Here's how the part is built. I have some questions about the finished solid (model axes, mm). Coordinates: 2 decimals unless noted, no trailing zeros. Write each loop counter-clockwise with the first axis right and the second up, starting at its lowest first coordinate (ties: lowest second). Pieces come first, ordered by that corner, then holes.
```python
from build123d import *

# Parameters (mm, degrees)
F1_DEPTH = 1
F2_R     = 2
F3_R     = 2.4
F4_DEPTH = 25
F5_R     = 2


with BuildPart() as f1:
    # F0 (on Front) → F1 (new body, symmetric)
    with BuildSketch(Plane.XZ):
        with BuildLine():
            ThreePointArc((28.013159, -35.217367), (14.836079, -42.484006), (0, -45))
            ThreePointArc((0, -45), (-14.836079, -42.484006), (-28.013159, -35.217367))
            Line((-28.013159, -35.217367), (-35, -44.00103))
            Line((-35, -44.00103), (-35, -65))
            Line((-35, -65), (35, -65))
            Line((35, -65), (35, -44.00103))
            Line((35, -44.00103), (28.013159, -35.217367))
        make_face()
        with BuildLine():
            ThreePointArc((0, -50), (-15.45085, -47.552826), (-29.389263, -40.45085))
            Line((-29.389263, -40.45085), (-27.038122, -37.214782))
            ThreePointArc((-27.038122, -37.214782), (-14.214782, -43.7486), (0, -46))
            ThreePointArc((0, -46), (14.214782, -43.7486), (27.038122, -37.214782))
            Line((27.038122, -37.214782), (29.389263, -40.45085))
            ThreePointArc((29.389263, -40.45085), (15.45085, -47.552826), (0, -50))
        make_face(mode=Mode.SUBTRACT)
    extrude(amount=F1_DEPTH, both=True)

    # F2
    f2_edges = [f1.edges().sort_by_distance(p)[0] for p in [
        (28.013159, 0, -35.217367),
        (35, 0, -44.00103),
        (-28.013159, 0, -35.217367),
        (-35, 0, -44.00103),
    ]]
    fillet(f2_edges, radius=F2_R)

    # F3 (on face) → F4 (cut)
    with BuildSketch(Plane.XZ.offset(1)):
        with Locations((-25, -55)):
            Circle(F3_R)
        with Locations((25, -55)):
            Circle(F3_R)
    extrude(amount=-F4_DEPTH, mode=Mode.SUBTRACT)

    # F5
    f5_edges = [f1.edges().sort_by_distance(p)[0] for p in [
        (35, 0, -65),
        (-35, 0, -65),
    ]]
    fillet(f5_edges, radius=F5_R)


solid = f1.part
```
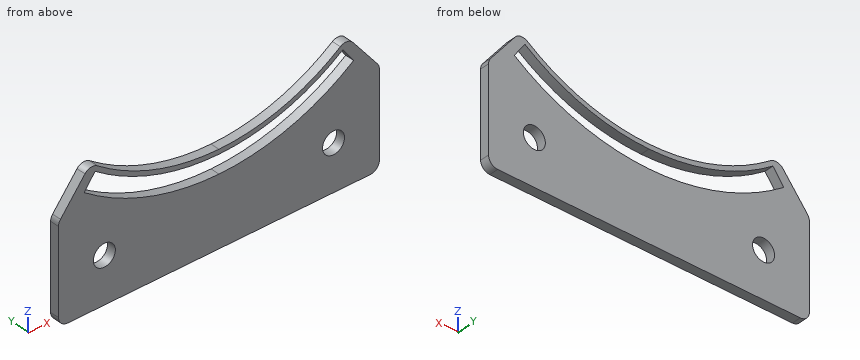
1) Imagine slicing it at A-A on z = -55. Please give me the cut outline in (x, y), then the cut area to 3 significant figures.
Values follow:
outline: (-35, -1) - (-27.4, -1) - (-27.4, 1) - (-35, 1) - close; (-22.6, -1) - (22.6, -1) - (22.6, 1) - (-22.6, 1) - close; (27.4, -1) - (35, -1) - (35, 1) - (27.4, 1) - close
area: 121 mm2
2) Will these pins go through, and if not, where does the flat tip stop? pin 1 (5.5 mm diameter, centred on x = -25, z = -55, fed in from -Y); pin 2 (1 mm diameter, centred on y = 0.5, z = -41, fed in from -X).
Values follow:
pin 1: stops at y = -1
pin 2: stops at x = -33.01
3) I need wall thicknesses on probe 1 along Z at (x, y) = (27, 0.2); probe 2 along X at (y, z) = (-0.45, -53.75); probe 3 along Z at (x, y) = (25, 0). Which ranges of each line are inside material? Lowest first, please.
Values follow:
probe 1: z = -65 to -56.33, -53.67 to -42.08, -37.24 to -36.11
probe 2: x = -35 to -27.05, -22.95 to 22.95, 27.05 to 35
probe 3: z = -65 to -57.4, -52.6 to -43.3, -38.61 to -37.42
4) Imagine slicing it at B-B on x = -2. Please give me the cut outline in (y, z).
Values follow:
outline: (-1, -65) - (1, -65) - (1, -49.96) - (-1, -49.96) - close; (-1, -45.96) - (1, -45.96) - (1, -44.96) - (-1, -44.96) - close
5) Imagine slicing it at D-D on x = -25. Please give me the cut outline in (y, z).
Values follow:
outline: (-1, -65) - (1, -65) - (1, -57.4) - (-1, -57.4) - close; (-1, -52.6) - (1, -52.6) - (1, -43.3) - (-1, -43.3) - close; (-1, -38.61) - (1, -38.61) - (1, -37.42) - (-1, -37.42) - close
6) Imagine slicing it at C-C on y = -0.7. Please give me the cut outline in (x, z).
Values follow:
outline: (-35, -63) arc R2 ccw to (-33, -65) - (33, -65) arc R2 ccw to (35, -63) - (35, -44.7) arc R2 ccw to (34.57, -43.45) - (29.23, -36.75) arc R2 ccw to (26.49, -36.38) arc R45 cw to (-26.49, -36.38) arc R2 ccw to (-29.23, -36.75) - (-34.57, -43.45) arc R2 ccw to (-35, -44.7) - close; hole (-29.39, -40.45) arc R50 ccw to (0, -50) arc R50 ccw to (29.39, -40.45) - (27.04, -37.21) arc R46 cw to (0, -46) arc R46 cw to (-27.04, -37.21) - close; hole circle Ø4.8 at (-25, -55); hole circle Ø4.8 at (25, -55)
